Verification items for this drawing (mm, ordinates from the low corner). A direction names the side the tool comes from. Coordinates: 2 decimals unless noted, no trailing zeros. Order: outer loops, then holes, each group sorted by start corner. A loop starts at its lowest first (then second) coordinate and runs counter-clockwise, first axis right, second up. Notation, with made-up numbers: (34.25, 34) - (67.25, 34) arc R14 ccw to (67.25, 56) - close; hole circle Ø7 at (63.25, 63). An arc over 180 degrees is marked (long way). One line per question, with ' | ' between items. Start each with the question number.
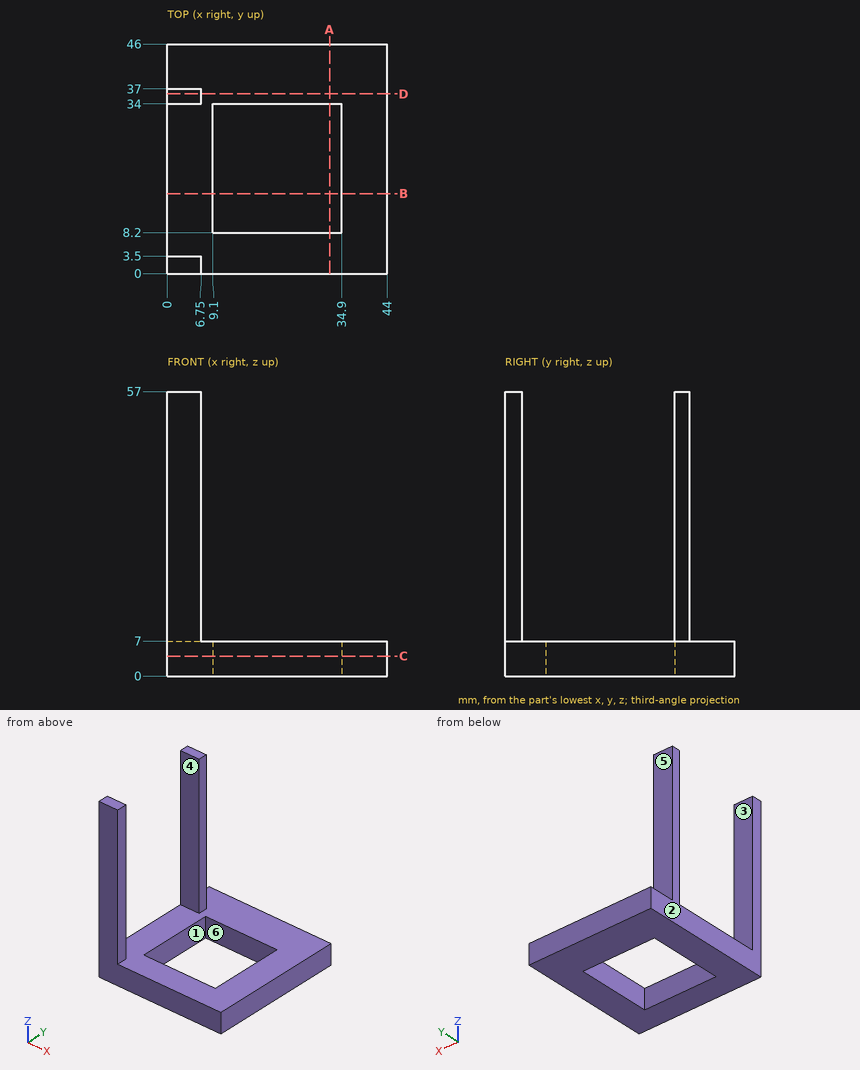
Item 1: Mould release check, pull along X, two halves, no side actions. Record for the marked faces 1, 2 and 3: +X half, -X half, draft (parallel to the pull), parting line (faces both ways), or undercut.
Item 2: Thickness scan on probe 1 along Y at (x, z) = (6.5, 19.5); probe 2 along Z at (x, y) = (31, 42). Record the ranges inside material, lowest first. Write a range as from..to.
Item 3: Section check D-D (y = 36). Record the cut outline in (x, z).
Item 4: Section check B-B (y = 16). Record the cut outline in (x, z).
Item 5: Gauge pin test, flat ends, axial feed: pin 1 (1.5 mm diameter, centred on x = 27, z = 8.5, fed in from +Y); pin 2 (3.5 mm diameter, centred on y = 36, z = 40, fed in from +X); pin 3 (5.5 mm diameter, centred on x = 5, z = 25.5, fed in from +Y); pin 4 (1.5 mm diameter, centred on x = 36, y = 7.5, fed in from +Z). Record the tip position at first contact, or that the pin passes through.
Item 6: Section check A-A (x = 32.5). Record the cut outline in (y, z).
Item 7: Set-up check for the marked faces 4, 5 and 6: record each of +Z, -Z, +X, -X, +Y, -Y from which the full face is reachable in a straight line by a thin tool's end or side.
Item 8: Section check C-C (z = 4). Record the cut outline in (x, y), then the cut area to 3 significant figures.
Completed:
1) face 1: undercut | face 2: -X half | face 3: draft
2) probe 1: y = 0..3.5, 34..37 | probe 2: z = 0..7
3) outline: (0, 0) - (44, 0) - (44, 7) - (6.75, 7) - (6.75, 57) - (0, 57) - close
4) outline: (0, 0) - (9.1, 0) - (9.1, 7) - (0, 7) - close; (34.9, 0) - (44, 0) - (44, 7) - (34.9, 7) - close
5) pin 1: passes through | pin 2: stops at x = 6.75 | pin 3: stops at y = 37 | pin 4: stops at z = 7
6) outline: (0, 0) - (8.2, 0) - (8.2, 7) - (0, 7) - close; (34, 0) - (46, 0) - (46, 7) - (34, 7) - close
7) face 4: +Z, +X, -X | face 5: +Z, +X, -X, +Y | face 6: +Z, -Z
8) outline: (0, 0) - (44, 0) - (44, 46) - (0, 46) - close; hole (9.1, 8.2) - (34.9, 8.2) - (34.9, 34) - (9.1, 34) - close | area: 1,360 mm^2
